CAD build for the part. Positions are in the model's coordinates, mm. Give positions to 0.01 mm unless a question says otherwise; leave off trailing zeros. Write each loop counter-clockwise with the first axis right and the second up, starting at its lowest first coordinate (ties: lowest second). Pieces come first, ordered by that corner, then holes. Notation, with made-up numbers: (48.25, 14) - (95.25, 14) arc R22 cw to (95.25, 23) - close; hole circle Ø6 at (86, 46). An arc over 180 degrees is marked (long way). Answer as a JSON object with one key per item and string values.
Autodesk Inventor part; units mm, degrees
ref_plane "YZ Plane" through (0, 0, 0) normal (1, 0, 0) x (0, 1, 0)
ref_plane "XZ Plane" through (0, 0, 0) normal (0, 1, 0) x (-1, 0, 0)
ref_plane "XY Plane" through (0, 0, 0) normal (0, 0, 1) x (1, 0, 0)
sketch "Skizze2" plane through (0, 0, 0) normal (0, 0, 1) x (1, 0, 0)
  circle A0 centre (0, 0) radius 67.5
  line L0 (-41.4214, 100) -> (41.4214, 100)
  line L1 (41.4214, 100) -> (100, 41.4214)
  line L2 (100, 41.4214) -> (100, -41.4214)
  line L3 (100, -41.4214) -> (41.4214, -100)
  line L4 (41.4214, -100) -> (-41.4214, -100)
  line L5 (-41.4214, -100) -> (-100, -41.4214)
  line L6 (-100, -41.4214) -> (-100, 41.4214)
  line L7 (-100, 41.4214) -> (-41.4214, 100)
  dimension "d6" = 135
  dimension "d10" = 200
extrude "Extrusion2" add sketch "Skizze2" along normal blind 15
equation "\"kg_thickness\" = 4.9"
equation "\"ht_thickness\" = 1.9"
equation "\"case_thickness\" = 18"
equation "\"inner_thickness\" = 15"
equation "\"gap_fit\" = 0.1"
equation "\"gap_slide\" = 0.2"
equation "\"gap_air\" = 1"
equation "\"bore_diameter\" = 73"
equation "\"mdf_thickness\" = 6"
equation "\"tape_width\" = 15"
equation "\"tape_thickness\" = 3"
equation "\"inner_depth\" = 255"
properties part number "Korpus_Motor_15mm"
(1) Flat gauge pin, fed straight in: P1, Ø8, axis at x = 50, z = 11.5, coming from the -Y side. Where does the tip first touch, or does it go through?
Answer key:
{"P1": "stops at y = -95.42"}
(2) Pull direction X, two halves, no side cores. Call faces 1 (the face through (-71.12, 70.3, 7.4)), 2 (the face through (-53.57, 41.07, 7.4)), 3 (the face through (100, 1, 7)), 4 (the face through (1, -100, 7)): pulls with the +X half, pulls with the -X half, needs draft (parallel to the pull), parting line crosses it, or undercut.
Answer key:
{"face 1": "pulls with the -X half", "face 2": "undercut", "face 3": "pulls with the +X half", "face 4": "needs draft"}
(3) Probe L1, parallel to Y at x = 0, z = 3; L2, parallel to X at y = 21, z = 12; L3, parallel to Y at x = 4, z = 9.5. List the from-to ranges inside material, lowest first. Write a range as [from, to].
Answer key:
{"L1": "y = [-100, -67.5], [67.5, 100]", "L2": "x = [-100, -64.15], [64.15, 100]", "L3": "y = [-100, -67.38], [67.38, 100]"}
(4) Saw through at B-B, the plane z = 5.25. Give the cut face in (x, y), and give its area (3 significant figures).
Answer key:
{"outline": "(-100, -41.42) - (-41.42, -100) - (41.42, -100) - (100, -41.42) - (100, 41.42) - (41.42, 100) - (-41.42, 100) - (-100, 41.42) - close; hole circle Ø135 at (0, 0)", "area": "18,800 mm²"}
(5) Saw through at D-D, the plane x = -86. Give the cut face in (y, z).
Answer key:
{"outline": "(-55.42, 0) - (55.42, 0) - (55.42, 15) - (-55.42, 15) - close"}
(6) Saw through at A-A, the plane y = 0. Give the cut face in (x, z), and give its area (3 significant figures).
Answer key:
{"outline": "(-100, 0) - (-67.5, 0) - (-67.5, 15) - (-100, 15) - close; (67.5, 0) - (100, 0) - (100, 15) - (67.5, 15) - close", "area": "975 mm²"}
